```python
from build123d import *

# Parameters (mm, degrees)
F0_W     = 152.4
F0_H     = 19.05
F1_DEPTH = 3.175
F2_R     = 2.54
F3_DEPTH = 3.176
F4_R     = 5.08
F5_R     = 2.54
F5_R_2   = 1.5875
F6_DEPTH = 3.176


with BuildPart() as f1:
    # F0 (on Top) → F1 (new body)
    with BuildSketch(Plane.XY):
        Rectangle(F0_W, F0_H)
    extrude(amount=F1_DEPTH)

    # F2 (on face) → F3 (cut, through all)
    with BuildSketch(Plane.XY.offset(3.175)):
        with Locations((-71.12, 4.7625)):
            Circle(F2_R)
        with Locations((-71.12, -4.7625)):
            Circle(F2_R)
        with Locations((71.12, 4.7625)):
            Circle(F2_R)
        with Locations((71.12, -4.7625)):
            Circle(F2_R)
    extrude(amount=-F3_DEPTH, mode=Mode.SUBTRACT)

    # F4
    f4_edges = [f1.edges().sort_by_distance(p)[0] for p in [
        (-76.2, 9.525, 1.5875),
        (-76.2, -9.525, 1.5875),
        (76.2, 9.525, 1.5875),
        (76.2, -9.525, 1.5875),
    ]]
    fillet(f4_edges, radius=F4_R)

    # F5 (on face) → F6 (cut, through all)
    with BuildSketch(Plane.XY.offset(3.175)):
        Circle(F5_R)
        with Locations((-4.7625, 0)):
            Circle(F5_R_2)
        with Locations((4.7625, 0)):
            Circle(F5_R_2)
    extrude(amount=-F6_DEPTH, mode=Mode.SUBTRACT)


solid = f1.part
```
Design review of the part built by this model. Coordinates are the model's own, in mm. Coordinates: 2 decimals unless noted, no trailing zeros. Order: outer loops, then holes, each group sorted by start corner. A loop starts at its lowest first (then second) coordinate and runs counter-clockwise, first axis right, second up.
1) Take a section at C-C, the plane y = -6. Give the boundary of the cut face in (x, z) (3 decimals).
2) Mouldability with a two-part tool opening along Y and no side actions: class faces 1 (the cylindrical face through (-0.33, 2.52, 1.61)), 2 (the cylindrical face through (74.67, -8.08, 1.61)), 3 (the flat face through (-1, 4, 3.175)) as +Y half, -Y half, draft (parallel to the pull), parting line (faces both ways), or undercut.
3) Clearance check with a flat-ended pin moving along its axis: pin 1 (4.5 mm diameter, centred on x = 0, y = 0, fed in from +Z). State where the tip first meets the part, or that it passes through.
4) Wall thickness on line 1 along Y through (x, z) = (71.12, 1.55) (1 decimal); line 2 along X through (y, z) = (-5, 1.8); line 3 along X through (y, z) = (4, 1.35): over which ranges is each line inside the solid? List them lowest first.
5) Take a section at A-A, the plane y = 0. Give the boundary of the cut face in (x, z) (3 decimals), and give its area (3 significant figures).
6) Take a section at B-B, the plane z = 1.7. State how many separate pieces and enclosed holes the cut face has, and give its area (3 significant figures).
Returned:
1. outline: (-75.956, 0) - (-73.338, 0) - (-73.338, 3.175) - (-75.956, 3.175) - close; (-68.902, 0) - (68.902, 0) - (68.902, 3.175) - (-68.902, 3.175) - close; (73.338, 0) - (75.956, 0) - (75.956, 3.175) - (73.338, 3.175) - close
2. face 1: undercut
2. face 2: -Y half
2. face 3: draft
3. pin 1: passes through
4. line 1: y = -9.5 to -7.3, -2.2 to 2.2, 7.3 to 9.5
4. line 2: x = -76.17 to -73.65, -68.59 to 68.59, 73.65 to 76.17
4. line 3: x = -76.2 to -73.54, -68.7 to 68.7, 73.54 to 76.2
5. outline: (-76.2, 0) - (-6.35, 0) - (-6.35, 3.175) - (-76.2, 3.175) - close; (-3.175, 0) - (-2.54, 0) - (-2.54, 3.175) - (-3.175, 3.175) - close; (2.54, 0) - (3.175, 0) - (3.175, 3.175) - (2.54, 3.175) - close; (6.35, 0) - (76.2, 0) - (76.2, 3.175) - (6.35, 3.175) - close
5. area: 448 mm2
6. separate pieces: 1
6. enclosed holes: 7
6. area: 2,760 mm2
